```python
from build123d import *

# Parameters (mm, degrees)
SKETCH1_R           = 12
SKETCH1_R_2         = 2.5
BOSS_EXTRUDE1_DEPTH = 1.2
SKETCH2_R           = 1.5
CUT_EXTRUDE1_DEPTH  = 1.2
SKETCH3_R           = 6.25
BOSS_EXTRUDE2_DEPTH = 12.3
SKETCH4_R           = 7
BOSS_EXTRUDE3_DEPTH = 12


with BuildPart() as part:
    # Sketch1 → Boss-Extrude1 (new body)
    with BuildSketch(Plane(origin=(0, 0, 0), x_dir=(1, 0, 0), z_dir=(0, 1, 0))):
        with Locations(Location((0, 0, 0), (0, 0, 270))):
            Circle(SKETCH1_R)
        with Locations(Location((0, 0, 0), (0, 0, 270))):
            Circle(SKETCH1_R_2, mode=Mode.SUBTRACT)
    extrude(amount=BOSS_EXTRUDE1_DEPTH)

    # Sketch2 → Cut-Extrude1 (cut)
    with BuildSketch(Plane(origin=(0, 1.2, 0), x_dir=(1, 0, 0), z_dir=(0, 1, 0))):
        with Locations(Location((0, 9.034469011, 0), (0, 0, 270))):
            Circle(SKETCH2_R)
        with Locations(Location((7.824079673, -4.517234506, 0), (0, 0, 270))):
            Circle(SKETCH2_R)
        with Locations(Location((-7.824079673, -4.517234506, 0), (0, 0, 270))):
            Circle(SKETCH2_R)
    extrude(amount=-CUT_EXTRUDE1_DEPTH, mode=Mode.SUBTRACT)

    # Sketch3 → Boss-Extrude2 (add)
    with BuildSketch(Plane(origin=(0, 0, 0), x_dir=(-1, 0, 0), z_dir=(0, -1, 0))):
        with Locations(Location((0, 0, 0), (0, 0, 270))):
            Circle(SKETCH3_R)
    extrude(amount=BOSS_EXTRUDE2_DEPTH)

    # Sketch4 → Boss-Extrude3 (add)
    with BuildSketch(Plane(origin=(0, 0, 0), x_dir=(1, 0, 0), z_dir=(0, 1, 0))):
        with Locations(Location((0, 0, 0), (0, 0, 270))):
            Circle(SKETCH4_R)
    extrude(amount=BOSS_EXTRUDE3_DEPTH)


solid = part.part
```
Design review of the part built by this model. Coordinates are the model's own, in mm. A direction names the side the tool comes from. Give positions to 0.01 mm unless a question says otherwise; leave off trailing zeros. Loops run counter-clockwise (first coordinate to the right, second up) from the corner with the lowest first, then second, coordinate; pieces in that order, holes last. Notation, with made-up numbers: (42.25, 49) -> (100.25, 49) arc R12 cw to (100.25, 72) -> close; hole circle Ø5 at (80.25, -20). An arc over 180 degrees is marked (long way). One line per item, written item: value.
Q1. For L1, parallel to Y at x = -8.25, z = -6.75; L2, parallel to Z at x = -0.25, y = -10 (3 decimals); L3, parallel to Z at x = 0.25, y = 3, list the stretches that pass through material, from the lowest coordinate up.
Numbers:
L1: y = 0 to 1.2
L2: z = -6.245 to 6.245
L3: z = -7 to 7
Q2. Machinability: for faces 1 (the cylindrical face through (-1.88, -6.06, 5.96)), 2 (the flat face through (0, -12.3, 0)), 3 (the flat face through (-5.2, 1.2, 5.2)), which of the approach directions +Z, -Z, +X, -X, +Y, -Y give a long, thin tool a straight path to every point of the face, cutting with its end or side? Answer none if there is none.
Numbers:
face 1: -Y
face 2: +Z, -Z, +X, -X, -Y
face 3: +Y
Q3. We need section D-D on z = 4.5. Give the boundary of the cut face in (x, y), and give its area (3 significant figures).
Numbers:
outline: (-11.12, 0) -> (-9.32, 0) -> (-9.32, 1.2) -> (-11.12, 1.2) -> close; (-6.32, 0) -> (-4.34, 0) -> (-4.34, -12.3) -> (4.34, -12.3) -> (4.34, 0) -> (6.32, 0) -> (6.32, 1.2) -> (5.36, 1.2) -> (5.36, 12) -> (-5.36, 12) -> (-5.36, 1.2) -> (-6.32, 1.2) -> close; (9.32, 0) -> (11.12, 0) -> (11.12, 1.2) -> (9.32, 1.2) -> close
area: 242 mm^2
Q4. For pin 1 Ø12 at (x, y) = (5, -9.5) entering from -Z; pin 2 Ø5 at (y, z) = (-2, -4) entering from -X; pin 3 Ø4 at (x, z) = (-6, -8.5) entering from +Y, all flat-tipped, find the tip position at first contact; note any pin that passes through.
Numbers:
pin 1: stops at z = -6.25
pin 2: stops at x = -11.74
pin 3: stops at y = 1.2
Q5. Draft analysis for pull direction Z (two halves, no side actions). For faces 4 (the cylindrical face through (-6.834, 6.524, -1.517)), 5 (the cylindrical face through (9.09, 0.61, 5.32)), 6 (the flat face through (-5, 0, 5)), state which applies: pulls with the +Z half, pulls with the -Z half, needs draft (parallel to the pull), parting line crosses it, or undercut.
Numbers:
face 4: parting line crosses it
face 5: undercut
face 6: needs draft
Q6. We need section C-C on y = 9. Give the boundary of the cut face in (x, z).
Numbers:
outline: circle Ø14 at (0, 0)
Q7. We need section B-B on z = 0. Give the boundary of the cut face in (x, y).
Numbers:
outline: (-12, 0) -> (-6.25, 0) -> (-6.25, -12.3) -> (6.25, -12.3) -> (6.25, 0) -> (12, 0) -> (12, 1.2) -> (7, 1.2) -> (7, 12) -> (-7, 12) -> (-7, 1.2) -> (-12, 1.2) -> close
Q8. We need section A-A on x = 0. Give the boundary of the cut face in (y, z), and give its area (3 significant figures).
Numbers:
outline: (-12.3, -6.25) -> (0, -6.25) -> (0, -7.53) -> (1.2, -7.53) -> (1.2, -7) -> (12, -7) -> (12, 7) -> (1.2, 7) -> (1.2, 12) -> (0, 12) -> (0, 6.25) -> (-12.3, 6.25) -> close; (0, -12) -> (1.2, -12) -> (1.2, -10.53) -> (0, -10.53) -> close
area: 330 mm^2
